from build123d import *

# Parameters (mm, degrees)
ESBO_O1_W                  = 14
ESBO_O1_H                  = 4.7
RESSALTO_EXTRUS_O1_DEPTH   = 3.05
CASCA1_T                   = -0.6
ESBO_O2_W                  = 8.1
ESBO_O2_H                  = 4.4
ESBO_O2_W_2                = 1.1
ESBO_O2_H_2                = 1.8
CORTE_EXTRUS_O1_DEPTH      = 0.6
ESBO_O3_W                  = 12.8
ESBO_O3_H                  = 3.5
RESSALTO_EXTRUS_O2_DEPTH   = 1.1
ESBO_O4_W                  = 14
ESBO_O4_H                  = 0.6
CORTE_EXTRUS_O2_DEPTH      = 0.8
CORTE_EXTRUS_O3_DEPTH      = 15.519814048
CORTE_EXTRUS_O3_DEPTH_BACK = 15.519814048
ESBO_O5_W                  = 0.9
ESBO_O5_H                  = 1.275071612
ESBO_O8_W                  = 0.5
ESBO_O8_H                  = 0.5
CORTE_EXTRUS_O5_DEPTH      = 10.577708494
ESBO_O9_W                  = 1.8
ESBO_O9_H                  = 4.707525417
ESBO_O9_H_2                = 4.692474583
CORTE_EXTRUS_O6_DEPTH      = 0.5
ESBO_O10_W                 = 1.8
ESBO_O10_H                 = 0.5
CORTE_EXTRUS_O7_DEPTH      = 9.962244011


with BuildPart() as part:
    # Esboço1 → Ressalto-extrusão1 (new, symmetric)
    with BuildSketch(Plane(origin=(0, 0, 0), x_dir=(1, 0, 0), z_dir=(0, 1, 0))):
        Rectangle(ESBO_O1_W, ESBO_O1_H)
    extrude(amount=RESSALTO_EXTRUS_O1_DEPTH, both=True)

    # Casca1
    casca1_openings = [part.faces().sort_by_distance(p)[0] for p in [
        (0, 3.05, 0),
    ]]
    offset(amount=CASCA1_T, openings=casca1_openings, kind=Kind.INTERSECTION)

    # Esboço2 → Corte-extrusão1 (cut)
    with BuildSketch(Plane(origin=(0, 0, -2.35), x_dir=(-1, 0, 0), z_dir=(0, 0, -1))):
        with Locations((0, 0.85)):
            Rectangle(ESBO_O2_W, ESBO_O2_H)
        with Locations((5.3, 0.15)):
            Rectangle(ESBO_O2_W_2, ESBO_O2_H_2)
        with Locations((-5.3, 0.15)):
            Rectangle(ESBO_O2_W_2, ESBO_O2_H_2)
    extrude(amount=-CORTE_EXTRUS_O1_DEPTH, mode=Mode.SUBTRACT)

    # Esboço3 → Ressalto-extrusão2 (add)
    with BuildSketch(Plane(origin=(0, -2.45, 0), x_dir=(1, 0, 0), z_dir=(0, 1, 0))):
        Rectangle(ESBO_O3_W, ESBO_O3_H)
    extrude(amount=RESSALTO_EXTRUS_O2_DEPTH)

    # Esboço4 → Corte-extrusão2 (cut)
    with BuildSketch(Plane(origin=(0, 0, -2.35), x_dir=(-1, 0, 0), z_dir=(0, 0, -1))):
        with Locations((0, -1.95)):
            Rectangle(ESBO_O4_W, ESBO_O4_H)
    extrude(amount=-CORTE_EXTRUS_O2_DEPTH, mode=Mode.SUBTRACT)

    # Esboço5 → Corte-extrusão3 (cut, two sides: drawn at the far end of the back side and taken through both)
    with BuildSketch(Plane(origin=(7, 0, 0), x_dir=(0, 0, -1), z_dir=(1, 0, 0)).offset(-CORTE_EXTRUS_O3_DEPTH_BACK)):
        with Locations((0.4, 2.412464194)):
            Rectangle(ESBO_O5_W, ESBO_O5_H)
    extrude(amount=CORTE_EXTRUS_O3_DEPTH + CORTE_EXTRUS_O3_DEPTH_BACK, mode=Mode.SUBTRACT)

    # Esboço8 → Corte-extrusão5 (cut, through all)
    with BuildSketch(Plane.XZ.offset(3.05)):
        with Locations((-3, 0)):
            Rectangle(ESBO_O8_W, ESBO_O8_H)
        with Locations((-5, 0)):
            Rectangle(ESBO_O8_W, ESBO_O8_H)
        with Locations((-1, 0)):
            Rectangle(ESBO_O8_W, ESBO_O8_H)
        with Locations((1, 0)):
            Rectangle(ESBO_O8_W, ESBO_O8_H)
        with Locations((3, 0)):
            Rectangle(ESBO_O8_W, ESBO_O8_H)
        with Locations((5, 0)):
            Rectangle(ESBO_O8_W, ESBO_O8_H)
    extrude(amount=-CORTE_EXTRUS_O5_DEPTH, mode=Mode.SUBTRACT)

    # Esboço9 → Corte-extrusão6 (cut)
    with BuildSketch(Plane.XZ.offset(3.05)):
        with Locations((-4.999992921, 0.003762709)):
            Rectangle(ESBO_O9_W, ESBO_O9_H)
        with Locations((-2.999992921, 0.003762709)):
            Rectangle(ESBO_O9_W, ESBO_O9_H)
        with Locations((-0.999992921, 0.003762709)):
            Rectangle(ESBO_O9_W, ESBO_O9_H)
        with Locations((0.999992921, 0.003762709)):
            Rectangle(ESBO_O9_W, ESBO_O9_H)
        with Locations((2.999992921, 0.003762709)):
            Rectangle(ESBO_O9_W, ESBO_O9_H)
        with Locations((4.999992921, 0.003762709)):
            Rectangle(ESBO_O9_W, ESBO_O9_H_2)
    extrude(amount=-CORTE_EXTRUS_O6_DEPTH, mode=Mode.SUBTRACT)

    # Esboço10 → Corte-extrusão7 (cut, through all)
    with BuildSketch(Plane.XY.offset(-2.342474583)):
        with Locations((4.999992921, -2.8)):
            Rectangle(ESBO_O10_W, ESBO_O10_H)
    extrude(amount=-CORTE_EXTRUS_O7_DEPTH, mode=Mode.SUBTRACT)


solid = part.part
Read the model definition and answer for the solid it produces. Units are mm, in the model's axes. A direction names the side the tool comes from. Coordinates: 2 decimals unless noted, no trailing zeros. Order: outer loops, then holes, each group sorted by start corner. A loop starts at its lowest first (then second) coordinate and runs counter-clockwise, first axis right, second up. Notation, with made-up numbers: (-23, -28.75) - (-19, -28.75) arc R15 cw to (-19, -3.75) - close; hole circle Ø5 at (11, 22). An arc over 180 degrees is marked (long way). Use one line per item in the form item = value.
(1) For a pull along X with two mould halves and no side action, classify faces 4 (the face through (7, 0, 0)), 5 (the face through (-7, 0, 0)), 6 (the face through (0, 1, 1.75)), 7 (the face through (-5.2, 1.4, -1.75)) as pulls with the +X half, pulls with the -X half, needs draft (parallel to the pull), parting line crosses it, or undercut.
Computed values:
face_4 = pulls with the +X half
face_5 = pulls with the -X half
face_6 = undercut
face_7 = undercut
(2) Straight lines are drawn through the part: L1, parallel to X at y = 0, z = -1.8; L2, parallel to Z at x = 4.5, y = 1.25; L3, parallel to Y at x = -1.5, z = -1.6. For each, find the intervals that lie inside material, in ascending order.
Computed values:
L1 = -7 to -5.85, -4.75 to -4.05, 4.05 to 4.75, 5.85 to 7
L2 = -2.35 to -1.75, 1.75 to 2.35
L3 = -2.55 to -2.25, -1.65 to -1.35
(3) Which of the six approach directions +Z, -Z, +X, -X, +Y, -Y give full straight-line access (tool end or side, diameter ignored) to faces 1 (the face through (2.59, -2.55, 0.03)), 2 (the face through (6.4, -3.05, 0)), 3 (the face through (-6.4, 1, 0))?
Computed values:
face_1 = +Z, -Z, -Y
face_2 = +Z, -Z, +X, -X, -Y
face_3 = +Y
(4) Given pin 1 Ø0.6 at (x, z) = (2.5, -2) entering from -Y, flat-ended and moving along its own axis, determine where the tip first touches the part or whether it passes through.
Computed values:
pin_1 = -2.55
(5) Section D-D, the plane x = 4.5 is taken. Give the vertices of the cut face in (y, z), then the cut area to 3 significant figures.
Computed values:
outline = (-2.55, -2.35) - (-2.25, -2.35) - (-2.25, -1.55) - (-1.65, -1.55) - (-1.65, -2.35) - (3.05, -2.35) - (3.05, -1.75) - (-1.35, -1.75) - (-1.35, 1.75) - (3.05, 1.75) - (3.05, 2.35) - (-2.55, 2.35) - close
area = 10.4 mm²
(6) Section A-A, the plane y = -0.5 is taken. Give the vertices of the cut face in (x, z), then the cut area to 3 significant figures.
Computed values:
outline = (-7, -2.35) - (-5.85, -2.35) - (-5.85, -1.75) - (-6.4, -1.75) - (-6.4, 1.75) - (6.4, 1.75) - (6.4, -1.75) - (5.85, -1.75) - (5.85, -2.35) - (7, -2.35) - (7, 2.35) - (-7, 2.35) - close; (-4.75, -2.35) - (-4.05, -2.35) - (-4.05, -1.75) - (-4.75, -1.75) - close; (4.05, -2.35) - (4.75, -2.35) - (4.75, -1.75) - (4.05, -1.75) - close
area = 14.8 mm²
(7) Section B-B, the plane y = -2 is taken. Give the vertices of the cut face in (x, z).
Computed values:
outline = (-7, -1.55) - (7, -1.55) - (7, 2.35) - (-7, 2.35) - close; hole (-5.25, -0.25) - (-4.75, -0.25) - (-4.75, 0.25) - (-5.25, 0.25) - close; hole (-3.25, -0.25) - (-2.75, -0.25) - (-2.75, 0.25) - (-3.25, 0.25) - close; hole (-1.25, -0.25) - (-0.75, -0.25) - (-0.75, 0.25) - (-1.25, 0.25) - close; hole (0.75, -0.25) - (1.25, -0.25) - (1.25, 0.25) - (0.75, 0.25) - close; hole (2.75, -0.25) - (3.25, -0.25) - (3.25, 0.25) - (2.75, 0.25) - close; hole (4.75, -0.25) - (5.25, -0.25) - (5.25, 0.25) - (4.75, 0.25) - close
